from build123d import *

# Parameters (mm, degrees)
BOSS_EXTRUDE1_DEPTH = 7
FILLET1_R           = 2
FILLET2_R           = 2
SKETCH2_R           = 1.5
SKETCH2_R_2         = 1.1
BOSS_EXTRUDE2_DEPTH = 4
SKETCH3_R           = 1.5
SKETCH3_R_2         = 1.1
SKETCH3_W           = 4.5
SKETCH3_H           = 1.5
BOSS_EXTRUDE3_DEPTH = 4


with BuildPart() as part:
    # Sketch1 → Boss-Extrude1 (new body)
    with BuildSketch(Plane(origin=(0, 0, 0), x_dir=(1, 0, 0), z_dir=(0, 1, 0))):
        with BuildLine():
            Line((10, -9), (-10, -9))
            ThreePointArc((-10, -9), (-11.414213562, -8.414213562), (-12, -7))
            Line((-12, -7), (-12, 7))
            ThreePointArc((-12, 7), (-11.414213562, 8.414213562), (-10, 9))
            Line((-10, 9), (10, 9))
            ThreePointArc((10, 9), (11.414213562, 8.414213562), (12, 7))
            Line((12, 7), (12, -7))
            ThreePointArc((12, -7), (11.414213562, -8.414213562), (10, -9))
        make_face()
    extrude(amount=BOSS_EXTRUDE1_DEPTH)

    # Fillet1
    fillet1_edges = [part.edges().sort_by_distance(p)[0] for p in [
        (11.414213562, 7, 8.414213562),
        (12, 7, 0),
        (11.414213562, 7, -8.414213562),
        (0, 7, -9),
        (-11.414213562, 7, -8.414213562),
        (-12, 7, 0),
        (-11.414213562, 7, 8.414213562),
        (0, 7, 9),
    ]]
    fillet(fillet1_edges, radius=FILLET1_R)

    # Fillet2
    fillet2_edges = [part.edges().sort_by_distance(p)[0] for p in [
        (12, 0, 0),
        (11.414213562, 0, 8.414213562),
        (0, 0, 9),
        (-11.414213562, 0, 8.414213562),
        (-12, 0, 0),
        (-11.414213562, 0, -8.414213562),
        (0, 0, -9),
        (11.414213562, 0, -8.414213562),
    ]]
    fillet(fillet2_edges, radius=FILLET2_R)

    # Sketch2 → Boss-Extrude2 (add)
    # profile 1 of 3: a face of its own
    with BuildSketch(Plane(origin=(12, 0, 0), x_dir=(0, 0, -1), z_dir=(1, 0, 0))):
        with Locations(Location((0, 3.5, 0), (0, 0, 270))):
            Circle(SKETCH2_R)
        with Locations((0, 3.5)):
            Circle(SKETCH2_R_2, mode=Mode.SUBTRACT)
    # profile 2 of 3: a face of its own
    with BuildSketch(Plane(origin=(12, 0, 0), x_dir=(0, 0, -1), z_dir=(1, 0, 0))):
        with Locations(Location((5.1879565, 3.5, 0), (0, 0, 270))):
            Circle(SKETCH2_R)
        with Locations((5.1879565, 3.5)):
            Circle(SKETCH2_R_2, mode=Mode.SUBTRACT)
    # profile 3 of 3: a face of its own
    with BuildSketch(Plane(origin=(12, 0, 0), x_dir=(0, 0, -1), z_dir=(1, 0, 0))):
        with Locations(Location((-5.396168524, 3.5, 0), (0, 0, 270))):
            Circle(SKETCH2_R)
        with Locations((-5.396168524, 3.5)):
            Circle(SKETCH2_R_2, mode=Mode.SUBTRACT)
    extrude(amount=BOSS_EXTRUDE2_DEPTH)

    # Sketch3 → Boss-Extrude3 (add)
    # profile 1 of 3: a face of its own
    with BuildSketch(Plane.ZY.offset(12)):
        with Locations((5.5, 3.5)):
            Circle(SKETCH3_R)
        with Locations((5.5, 3.5)):
            Circle(SKETCH3_R_2, mode=Mode.SUBTRACT)
    # profile 2 of 3: a face of its own
    with BuildSketch(Plane.ZY.offset(12)):
        with Locations(Location((1.1, 3.5, 0), (0, 0, 270))):
            Circle(SKETCH3_R)
        with Locations((1.1, 3.5)):
            Circle(SKETCH3_R_2, mode=Mode.SUBTRACT)
    # profile 3 of 3: a face of its own
    with BuildSketch(Plane.ZY.offset(12)):
        with Locations((-3.974486265, 3.5)):
            Rectangle(SKETCH3_W, SKETCH3_H)
    extrude(amount=BOSS_EXTRUDE3_DEPTH)


solid = part.part
For this review, take the finished solid that the model builds, in its own axes (mm). A direction names the side the tool comes from. Give positions to 0.01 mm unless a question says otherwise; leave off trailing zeros. Loops run counter-clockwise (first coordinate to the right, second up) from the corner with the lowest first, then second, coordinate; pieces in that order, holes last. Notation, with made-up numbers: M -18,54 L 18,54 A16 cw 18,73 Z; hole C -1.5,10.25 d8. An arc over 180 degrees is marked long. Put each result on its own line as item: value. Start each with the question number.
(1) For pin 1 (2 mm diameter, centred on x = -14.5, z = -5, fed in from -Y); pin 2 (0.7 mm diameter, centred on y = 4, z = 0, fed in from +X); pin 3 (1.8 mm diameter, centred on y = 3, z = -5, fed in from +X); pin 4 (1.6 mm diameter, centred on x = -14, y = 3.5, fed in from +Z), all flat-tipped, find the tip position at first contact; note any pin that passes through.
(2) Wall thickness on L1, parallel to Y at x = -14, z = 5.5; L2, parallel to X at y = 4.75, z = 1.25; L3, parallel to X at y = 3.5, z = 3: over which ranges is each line inside the solid? List them lowest first.
(3) The part is to be moulded in two halves that separate along Y. For faces 6 (the cylindrical face through (0.14, 0.57, -8.4)), 7 (the flat face through (-12, 3, 1)), 8 (the cylindrical face through (11.43, 6.4, 0.1)), say which applies: +Y half, -Y half, draft (parallel to the pull), parting line (faces both ways), or undercut.
(4) Machinability: for faces 1 (the flat face through (-14, 2.75, -4)), 2 (the flat face through (12, 3, -5)), 3 (the cylindrical face through (11.43, 3.48, 8.4)), 4 (the flat face through (-14, 3, -6.224)), 5 (the flat face through (-12, 3, 3)), which of the approach directions +Z, -Z, +X, -X, +Y, -Y give a long, thin tool a straight path to every point of the face, cutting with its end or side? Answer none if there is none.
(5) Add section D-D, the plane y = 1.25. Write out the cut boundary in (x, z).
(6) Add section A-A, the plane x = 13. Write out the cut boundary in (y, z).
(7) Add section C-C, the plane z = -4.5. Write out the cut boundary in (x, y), then the cut area to 3 significant figures.
(8) Add section B-B, the plane x = 1. Write out the cut boundary in (y, z).
Result:
1. pin 1: stops at y = 2.75
1. pin 2: stops at x = 12
1. pin 3: stops at x = 16
1. pin 4: stops at z = 7
2. L1: y = 2 to 2.4, 4.6 to 5
2. L2: x = -16 to 12
2. L3: x = -12 to 12
3. face 6: -Y half
3. face 7: undercut
3. face 8: +Y half
4. face 1: -Z, -X, -Y
4. face 2: +X
4. face 3: +Z, +X, +Y, -Y
4. face 4: -Z, -X, +Y, -Y
4. face 5: -X
5. outline: M -11.85,-7 A1.85 ccw -10,-8.85 L 10,-8.85 A1.85 ccw 11.85,-7 L 11.85,7 A1.85 ccw 10,8.85 L -10,8.85 A1.85 ccw -11.85,7 Z
6. outline: C 3.5,-5.19 d3; C 3.5,0 d3; C 3.5,5.4 d3; hole C 3.5,-5.19 d2.2; hole C 3.5,0 d2.2; hole C 3.5,5.4 d2.2
7. outline: M -16,2.75 L -12,2.75 L -12,2 A2 ccw -10,0 L 10,0 A2 ccw 12,2 L 12,2.17 L 16,2.17 L 16,2.64 L 12,2.64 L 12,4.36 L 16,4.36 L 16,4.83 L 12,4.83 L 12,5 A2 ccw 10,7 L -10,7 A2 ccw -12,5 L -12,4.25 L -16,4.25 Z
7. area: 174 mm^2
8. outline: M 0,-7 A2 ccw 2,-9 L 5,-9 A2 ccw 7,-7 L 7,7 A2 ccw 5,9 L 2,9 A2 ccw 0,7 Z
